from build123d import *

# Parameters (mm, degrees)
SKETCH1_W            = 185
SKETCH1_H            = 160
BOSS_EXTRUDE1_DEPTH  = 20
SKETCH2_W            = 20
SKETCH2_H            = 160
BOSS_EXTRUDE2_DEPTH  = 180
SKETCH4_W            = 50
SKETCH4_H            = 50
CUT_EXTRUDE1_DEPTH   = 201
SKETCH3_W            = 20
SKETCH3_H            = 200
BOSS_EXTRUDE3_DEPTH  = 20
FILLET1_R            = 5
SKETCH6_W            = 8.2
SKETCH6_H            = 30.4
CUT_EXTRUDE2_DEPTH   = 12.5
FILLET2_R            = 5
FILLET2_OF_MIRROR1_R = 5
SKETCH7_W            = 165
SKETCH7_H            = 190
CUT_EXTRUDE3_DEPTH   = 12.5


with BuildPart() as part:
    # Sketch1 → Boss-Extrude1 (new body)
    with BuildSketch(Plane.XY):
        with Locations((92.5, 80)):
            Rectangle(SKETCH1_W, SKETCH1_H)
    extrude(amount=BOSS_EXTRUDE1_DEPTH)

    # Sketch2 → Boss-Extrude2 (add)
    with BuildSketch(Plane.XY.offset(20)):
        with Locations((10, 80)):
            Rectangle(SKETCH2_W, SKETCH2_H)
        with Locations((175, 80)):
            Rectangle(SKETCH2_W, SKETCH2_H)
    extrude(amount=BOSS_EXTRUDE2_DEPTH)

    # Sketch4 → Cut-Extrude1 (cut, through all)
    with BuildSketch(Plane(origin=(0, 0, 0), x_dir=(-1, 0, 0), z_dir=(0, 0, -1))):
        with Locations((-92.5, 25)):
            Rectangle(SKETCH4_W, SKETCH4_H)
    extrude(amount=-CUT_EXTRUDE1_DEPTH, mode=Mode.SUBTRACT)

    # Sketch3 → Boss-Extrude3 (add)
    with BuildSketch(Plane.XZ):
        with Locations((175, 100)):
            Rectangle(SKETCH3_W, SKETCH3_H)
    extrude(amount=BOSS_EXTRUDE3_DEPTH)

    # Fillet1
    fillet1_edges = [part.edges().sort_by_distance(p)[0] for p in [
        (67.5, 50, 10),
        (67.5, 0, 10),
        (117.5, 0, 10),
        (117.5, 50, 10),
        (165, 0, 10),
    ]]
    fillet(fillet1_edges, radius=FILLET1_R)

    # Sketch6 → Cut-Extrude2 (cut)
    with BuildSketch(Plane.XY.offset(200)):
        with Locations((10, 80)):
            Rectangle(SKETCH6_W, SKETCH6_H)
    cut_extrude2 = extrude(amount=-CUT_EXTRUDE2_DEPTH, mode=Mode.SUBTRACT)

    # Fillet2
    fillet2_edges = [part.edges().sort_by_distance(p)[0] for p in [
        (10, 64.8, 187.5),
        (10, 95.2, 187.5),
    ]]
    fillet(fillet2_edges, radius=FILLET2_R)

    # Mirror1: Cut-Extrude2 across plane
    add(cut_extrude2.mirror(Plane(origin=(92.5, 0, 0), x_dir=(0, 0, 1), z_dir=(1, 0, 0))), mode=Mode.SUBTRACT)

    # Fillet2 of Mirror1
    fillet2_of_mirror1_edges = [part.edges().sort_by_distance(p)[0] for p in [
        (175, 64.8, 187.5),
        (175, 95.2, 187.5),
    ]]
    fillet(fillet2_of_mirror1_edges, radius=FILLET2_OF_MIRROR1_R)

    # Sketch7 → Cut-Extrude3 (cut)
    with BuildSketch(Plane(origin=(0, 160, 0), x_dir=(1, 0, 0), z_dir=(0, 1, 0))):
        with Locations((92.5, -105)):
            Rectangle(SKETCH7_W, SKETCH7_H)
    extrude(amount=-CUT_EXTRUDE3_DEPTH, mode=Mode.SUBTRACT)


solid = part.part
CAD build for the part. Positions are in the model's coordinates, mm. A direction names the side the tool comes from. Coordinates: 2 decimals unless noted, no trailing zeros. Loops run counter-clockwise (first coordinate to the right, second up) from the corner with the lowest first, then second, coordinate; pieces in that order, holes last. Notation, with made-up numbers: (36.25, 5) -> (59.25, 5) arc R11 ccw to (59.25, 10) -> close; hole circle Ø2 at (69, -31.75). An arc over 180 degrees is marked (long way). One line per item, written item: value.
1. Which spindle directions (+Z, -Z, +X, -X, +Y, -Y) get a long thin tool onto all of the face, cutting with end or side? Do faces 4 (the face through (19, 147.5, 90)), 5 (the face through (141, 0, 10)), 6 (the face through (14.1, 80, 194)), 7 (the face through (91, 72, 20)). Say none if no direction does.
Answers:
face 4: +Z, +Y
face 5: +Z, -Z, -X, -Y
face 6: +Z
face 7: +Z, +Y, -Y
2. Slice it at D-D on z = 13.5. Write the cut outline in (x, y), and give its area (3 significant figures).
Answers:
outline: (0, 0) -> (62.5, 0) arc R5 ccw to (67.5, 5) -> (67.5, 45) arc R5 cw to (72.5, 50) -> (112.5, 50) arc R5 cw to (117.5, 45) -> (117.5, 5) arc R5 ccw to (122.5, 0) -> (160, 0) arc R5 cw to (165, -5) -> (165, -20) -> (185, -20) -> (185, 160) -> (175, 160) -> (175, 147.5) -> (10, 147.5) -> (10, 160) -> (0, 160) -> close
area: 25,400 mm^2
3. Slice it at A-A on z = 57.5. Write the cut outline in (x, y).
Answers:
outline: (0, 0) -> (20, 0) -> (20, 147.5) -> (10, 147.5) -> (10, 160) -> (0, 160) -> close; (165, -20) -> (185, -20) -> (185, 160) -> (175, 160) -> (175, 147.5) -> (165, 147.5) -> close
4. Slice it at B-B on y = 33. Write the cut outline in (x, z), and give its area (3 significant figures).
Answers:
outline: (0, 0) -> (67.5, 0) -> (67.5, 20) -> (20, 20) -> (20, 200) -> (0, 200) -> close; (117.5, 0) -> (185, 0) -> (185, 200) -> (165, 200) -> (165, 20) -> (117.5, 20) -> close
area: 9,900 mm^2
5. Flat gauge pins, fed straight in: P1, Ø10, axis at x = 78.5, y = 156.5, coming from the +Z side; P2, Ø4, axis at x = 174, y = 83, coming from the +Z side; P3, Ø5, axis at x = 148, z = 21, coming from the -Y side. Where does each tip first touch, or does it go through?
Answers:
P1: stops at z = 10
P2: stops at z = 187.5
P3: stops at y = 0
6. Pull direction X, two halves, no side cores. Call faces 1 (the face through (174.94, 93.77, 189)), 2 (the face through (5, 81, 200)), 3 (the face through (164, -2, 10)): pulls with the +X half, pulls with the -X half, needs draft (parallel to the pull), parting line crosses it, or undercut.
Answers:
face 1: undercut
face 2: needs draft
face 3: pulls with the -X half
7. Slice it at C-C on y = 75. Write the cut outline in (x, z), and give its area (3 significant figures).
Answers:
outline: (0, 0) -> (185, 0) -> (185, 200) -> (179.1, 200) -> (179.1, 187.5) -> (170.9, 187.5) -> (170.9, 200) -> (165, 200) -> (165, 20) -> (20, 20) -> (20, 200) -> (14.1, 200) -> (14.1, 187.5) -> (5.9, 187.5) -> (5.9, 200) -> (0, 200) -> close
area: 10,700 mm^2
8. Drill centre lines: line 1 (X direction, y = 95, z = 170.5); line 2 (Z direction, x = 122, y = 95.5); line 3 (X direction, y = 151, z = 34). Where is each one in solid material? Low to high. Write a range as [from, to].
Answers:
line 1: x = [0, 20], [165, 185]
line 2: z = [0, 20]
line 3: x = [0, 10], [175, 185]
